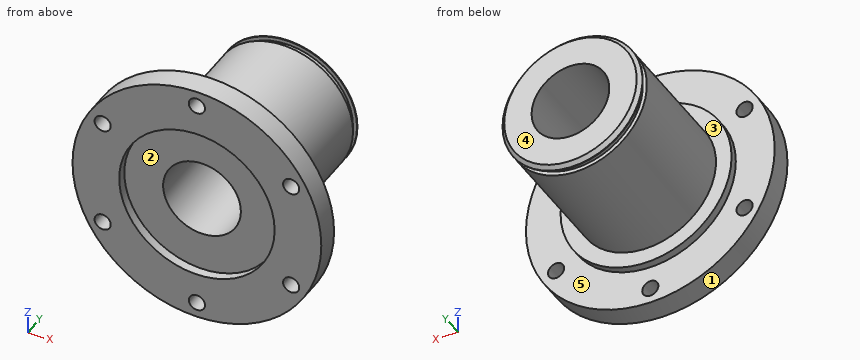
Autodesk Inventor part; units mm, degrees
ref_plane "YZ Plane" through (0, 0, 0) normal (1, 0, 0) x (0, 1, 0)
ref_plane "XZ Plane" through (0, 0, 0) normal (0, 1, 0) x (-1, 0, 0)
ref_plane "XY Plane" through (0, 0, 0) normal (0, 0, 1) x (1, 0, 0)
sketch "Sketch1" plane through (0, 0, 0) normal (0, 0, 1) x (1, 0, 0)
  line L0 (0, 0) -> (0, 30.8582)
  line L1 (7.9375, 1.905) -> (7.9375, 34.544)
  line L2 (7.9375, 34.544) -> (14.2875, 34.544)
  line L3 (14.2875, 34.544) -> (14.2875, 6.35)
  line L4 (17.4625, 4.7625) -> (25.4, 4.7625)
  line L5 (25.4, 4.7625) -> (25.4, 0)
  line L6 (25.4, 0) -> (15.875, 0)
  line L7 (7.9375, 1.905) -> (15.875, 1.905)
  line L8 (15.875, 1.905) -> (15.875, 0)
  line L9 (14.2875, 6.35) -> (17.4625, 6.35)
  line L10 (17.4625, 6.35) -> (17.4625, 4.7625)
  dimension "d0" = 50.8
  dimension "d1" = 15.875
  dimension "d2" = 28.575
  dimension "d3" = 4.7625
  dimension "d19" = 31.75
  dimension "d20" = 1.905
  dimension "d30" = 34.925
  dimension "d31" = 1.5875
  dimension "d34" = 34.544
revolve "Revolution1" add sketch "Sketch1" angle 360 about axis through (0, 0, 0) along (0, 1, 0)
sketch "Sketch4" plane through (0, 0, 0) normal (0, 0, 1) x (1, 0, 0)
  line L0 (13.4493, 33.6296) -> (17.9779, 33.6296)
  line L1 (17.9779, 33.6296) -> (17.9779, 32.131)
  line L2 (17.9779, 32.131) -> (13.4493, 32.131)
  line L3 (13.4493, 32.131) -> (13.4493, 33.6296)
  line L4 (-25.4, 4.7625) -> (25.4, 4.7625)
  line L5 (-14.2875, 34.544) -> (14.2875, 34.544)
  line L6 (0, 34.544) -> (0, 40.6447)
  line L7 (-17.4625, 6.35) -> (17.4625, 6.35)
  point P0 (0, 0)
  dimension "d26" = 1.4986
  dimension "d27" = 26.8986
  dimension "d33" = 25.781
revolve "Revolution2" cut sketch "Sketch4" angle 360 about axis through (0, 34.544, 0) along (0, 1, 0)
chamfer "Chamfer1" distance 0.762 angle 45 1 edges at (-14.2875, 34.544, 0)
sketch "Sketch2" plane through (0, 0, 0) normal (0, -1, 0) x (1, 0, 0)
  circle A0 centre (0, 0) radius 22.225 construction
  point P0 (0, -22.225)
  point P1 (19.2474, -11.1125)
  point P2 (19.2474, 11.1125)
  point P3 (0, 22.225)
  point P4 (-19.2474, 11.1125)
  point P5 (-19.2474, -11.1125)
  dimension "d7" = 44.45
  dimension "d10" = 360
hole "Hole1" at (0, 0, -22.225) at (19.2474, 0, -11.1125) at (19.2474, 0, 11.1125) at (0, 0, 22.225) at (-19.2474, 0, 11.1125) at (-19.2474, 0, -11.1125) direction (0, 1, 0) diameter 3.302 end through all
properties part number "FLY_006_HoodPivot" material "Aluminum 6061"
CAD build for the part. Positions are in the model's coordinates, mm. Face numbers are marked on the shaded views. A direction names the side the tool comes from. Give positions to 0.01 mm unless a question says otherwise; leave off trailing zeros. Order: outer loops, then holes, each group sorted by start corner. A loop starts at its lowest first (then second) coordinate and runs counter-clockwise, first axis right, second up. Notation, with made-up numbers: (55.5, 58) - (63.5, 58) arc R33 ccw to (63.5, 89) - close; hole circle Ø1 at (-36, 47). An arc over 180 degrees is marked (long way). Answer in a Markdown table with one row per item.
1. Saw through at B-B, the plane y = 10.5. Give the cut face in (x, z) (1 decimal), plus the area to 3 significant figures.
Data:
| item | result |
|---|---|
| outline | circle Ø28.6 at (0, 0); hole circle Ø15.9 at (0, 0) |
| area | 443 mm² |
2. Saw through at C-C, the plane x = 0. Count the separate pieces of the cut face and the enclosed holes in it, plus the area to 3 significant figures.
Data:
| item | result |
|---|---|
| separate pieces | 4 |
| enclosed holes | 0 |
| area | 490 mm² |
3. Flat gauge pins, fed straight in: pin 1 (8.5 mm diameter, centred on x = 1.5, z = 4, fed in from -Y) (3 decimals); pin 2 (10 mm diameter, centred on x = 15.5, y = 12, fed in from +Z); pin 3 (5.5 mm diameter, centred on x = 19.25, z = 11.11, fed in from +Y). Where does each tip first touch, or does it go through?
Data:
| item | result |
|---|---|
| pin 1 | stops at y = 1.905 |
| pin 2 | stops at z = 9.69 |
| pin 3 | stops at y = 4.76 |
4. Probe probe 1 along Z at (x, y) = (0, 3); probe 2 along Z at (x, y) = (0, 1.3) (3 decimals); probe 3 along X at (y, z) = (0.9, 0) (3 decimals). List the from-to ranges inside material, lowest first. Write a range as [from, to].
Data:
| item | result |
|---|---|
| probe 1 | z = [-25.4, -23.88], [-20.57, -7.94], [7.94, 20.57], [23.88, 25.4] |
| probe 2 | z = [-25.4, -23.876], [-20.574, -15.875], [15.875, 20.574], [23.876, 25.4] |
| probe 3 | x = [-25.4, -15.875], [15.875, 25.4] |
5. Tool access for the marked faces 4 and 5: list every direction of +Z, -Z, +X, -X, +Y, -Y with a clear straight run to the whole face (end or side of a thin tool).
Data:
| item | result |
|---|---|
| face 4 | +Z, -Z, +X, -X, +Y |
| face 5 | +Y |
6. Pull direction X, two halves, no side cores. Call the marked faces 1, 2 and 3: pulls with the +X half, pulls with the -X half, needs draft (parallel to the pull), parting line crosses it, or undercut.
Data:
| item | result |
|---|---|
| face 1 | parting line crosses it |
| face 2 | undercut |
| face 3 | needs draft |
